from build123d import *

# Parameters (mm, degrees)
PAD023_DEPTH    = 20
SKETCH041_R     = 3
POCKET012_DEPTH = 44.001
SKETCH042_R     = 3
POCKET013_DEPTH = 5
SKETCH044_W     = 44
SKETCH044_H     = 4
PAD025_DEPTH    = 20
SKETCH045_W     = 20
SKETCH045_H     = 10
SKETCH045_W_2   = 14
SKETCH045_H_2   = 4
PAD026_DEPTH    = 20
SKETCH046_R     = 1.4
POCKET014_DEPTH = 6.001


with BuildPart() as part:
    # Sketch040 → Pad023 (new body)
    with BuildSketch(Plane.XY):
        with BuildLine():
            Line((0, -44), (0, 0))
            Line((0, 0), (20, 0))
            Line((20, 0), (20, -5))
            Line((20, -5), (7, -5))
            ThreePointArc((7, -5), (4.87868, -5.87868), (4, -8))
            Line((4, -8), (4, -44))
            Line((4, -44), (0, -44))
        make_face()
    extrude(amount=PAD023_DEPTH)

    # Sketch041 → Pocket012 (cut, through all)
    with BuildSketch(Plane.XZ):
        with Locations((14, 5)):
            Circle(SKETCH041_R)
    extrude(amount=POCKET012_DEPTH, mode=Mode.SUBTRACT)

    # Sketch042 → Pocket013 (cut)
    with BuildSketch(Plane.YZ):
        with Locations((-38, 9)):
            Circle(SKETCH042_R)
    extrude(amount=POCKET013_DEPTH, mode=Mode.SUBTRACT)

    # Sketch044 → Pad025 (join)
    with BuildSketch(Plane.YZ):
        with Locations((-22, -2)):
            Rectangle(SKETCH044_W, SKETCH044_H)
    extrude(amount=PAD025_DEPTH)

    # Sketch045 → Pad026 (join)
    with BuildSketch(Plane.YZ):
        with Locations((-10.041618, -9)):
            Rectangle(SKETCH045_W, SKETCH045_H)
        with Locations((-10.041618, -9)):
            Rectangle(SKETCH045_W_2, SKETCH045_H_2, mode=Mode.SUBTRACT)
    extrude(amount=PAD026_DEPTH)

    # Sketch046 → Pocket014 (cut, through all)
    with BuildSketch(Plane.XY.offset(-8)):
        with Locations((10, -15)):
            Circle(SKETCH046_R)
        with Locations((10, -5)):
            Circle(SKETCH046_R)
    extrude(amount=-POCKET014_DEPTH, mode=Mode.SUBTRACT)


solid = part.part
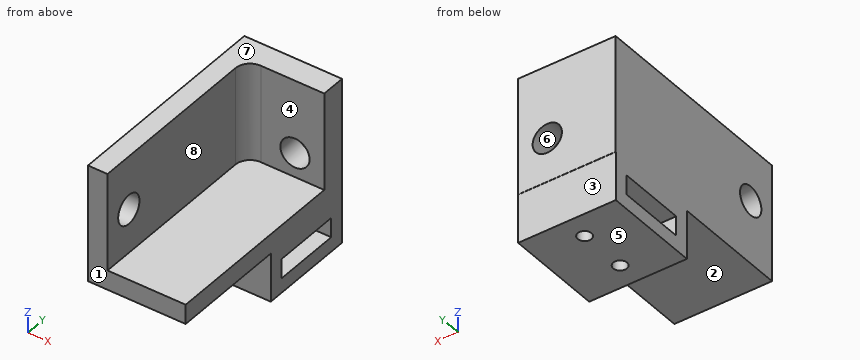
Read the model definition and answer for the solid it produces. Units are mm, in the model's axes. Face numbers are marked on the shaded views. A direction names the side the tool comes from. Coordinates: 2 decimals unless noted, no trailing zeros. Loops run counter-clockwise (first coordinate to the right, second up) from the corner with the lowest first, then second, coordinate; pieces in that order, holes last. Notation, with made-up numbers: (49.25, 70) -> (76.25, 70) arc R21 ccw to (76.25, 101) -> close; hole circle Ø9 at (-31, -11.75). An arc over 180 degrees is marked (long way). Answer in a Markdown table with one row per item.
Item 1: A cutting plane is placed at C-C on z = 5. Determine the outline of the cut face in (x, y), plus the area to 3 significant figures.
Returned:
| item | result |
|---|---|
| outline | (0, -44) -> (4, -44) -> (4, -8) arc R3 cw to (7, -5) -> (11, -5) -> (11, 0) -> (0, 0) -> close; (17, -5) -> (20, -5) -> (20, 0) -> (17, 0) -> close |
| area | 228 mm^2 |
Item 2: A cutting plane is placed at B-B on y = -38. Determine the outline of the cut face in (x, z), plus the area to 3 significant figures.
Returned:
| item | result |
|---|---|
| outline | (0, -4) -> (20, -4) -> (20, 0) -> (4, 0) -> (4, 6) -> (0, 6) -> close; (0, 12) -> (4, 12) -> (4, 20) -> (0, 20) -> close |
| area | 136 mm^2 |
Item 3: A cutting plane is placed at D-D on x = 2.75. Determine the outline of the cut face in (y, z).
Returned:
| item | result |
|---|---|
| outline | (-44, -4) -> (-20.04, -4) -> (-20.04, -14) -> (-0.04, -14) -> (-0.04, -4) -> (0, -4) -> (0, 20) -> (-44, 20) -> close; hole circle Ø6 at (-38, 9); hole (-17.04, -11) -> (-3.04, -11) -> (-3.04, -7) -> (-17.04, -7) -> close |
Item 4: For a pull along X with two mould halves and no side action, classify the marked faces 6, 7 and 8 as released by +X, released by -X, zero draft, split by the parting line, or undercut.
Returned:
| item | result |
|---|---|
| face 6 | undercut |
| face 7 | zero draft |
| face 8 | released by +X |
Item 5: A cutting plane is placed at A-A on x = 14. Determine the outline of the cut face in (y, z), plus the area to 3 significant figures.
Returned:
| item | result |
|---|---|
| outline | (-44, -4) -> (-20.04, -4) -> (-20.04, -14) -> (-0.04, -14) -> (-0.04, -4) -> (0, -4) -> (0, 2) -> (-5, 2) -> (-5, 0) -> (-44, 0) -> close; (-5, 8) -> (0, 8) -> (0, 20) -> (-5, 20) -> close; hole (-17.04, -11) -> (-3.04, -11) -> (-3.04, -7) -> (-17.04, -7) -> close |
| area | 390 mm^2 |
Item 6: Straight lines are drawn through the part: line 1 along Y through (x, z) = (10, -12.05); line 2 along X through (y, z) = (-1.6, 5); line 3 along Y through (x, z) = (10.5, -8.5). For each, find the intervals that lie inside material, in ascending order. Write a range as [from, to].
Returned:
| item | result |
|---|---|
| line 1 | y = [-20.04, -16.4], [-13.6, -6.4], [-3.6, -0.04] |
| line 2 | x = [0, 11], [17, 20] |
| line 3 | y = [-20.04, -17.04], [-3.04, -0.04] |
Item 7: For the marked faces 1, 2, 3, 4 and 5, determine the directions among +Z, -Z, +X, -X, +Y, -Y from which every point of the face is accessible in a straight line to the end or side of a thin tool.
Returned:
| item | result |
|---|---|
| face 1 | +Z, -Z, +X, -X, -Y |
| face 2 | -Z, +X, -X, -Y |
| face 3 | -Z, +X, -X, +Y |
| face 4 | +Z, +X, -Y |
| face 5 | -Z, +X, -X, +Y, -Y |
Item 8: Each of these flat-tipped pins is pushed along its axis until it touches: P1, Ø7, axis at x = 14.5, y = -9.5, coming from the +Z side; P2, Ø2, axis at x = 8, z = -9, coming from the +Y side; P3, Ø1, axis at x = 8, y = -25, coming from the -Z side. Where does it stop, or does it pass through?
Returned:
| item | result |
|---|---|
| P1 | stops at z = 0 |
| P2 | stops at y = -0.04 |
| P3 | stops at z = -4 |
